Here's how the part is built. I have some questions about the finished solid (model axes, mm). Face numbers are marked on the shaded views. A direction names the side the tool comes from. Round coordinates to 2 decimals unless told otherwise and drop trailing zeros. Loops run counter-clockwise (first coordinate to the right, second up) from the corner with the lowest first, then second, coordinate; pieces in that order, holes last. Notation, with made-up numbers: (62, -11.5) - (79, -11.5) arc R29 ccw to (79, 15.5) - close; hole circle Ø1 at (-40, -23). An arc over 180 degrees is marked (long way). Return JSON: item names as keys, results as strings. Group by question number.
```python
from build123d import *

# Parameters (mm, degrees)
F0_W      = 37
F0_H      = 15
F1_DEPTH  = 3.97
F2_W      = 17
F2_H      = 13.5
F3_DEPTH  = 13.5
F4_R      = 4.85
F5_DEPTH  = 15
F6_R      = 3.15
F7_DEPTH  = 22.001
F8_W      = 17
F8_H      = 7
F9_DEPTH  = 9
F10_R     = 1.55
F11_DEPTH = 11.001
F12_W     = 17
F12_H     = 3
F13_DEPTH = 17.5
F15_DEPTH = 3.971


with BuildPart() as f1:
    # F0 (on Top) → F1 (new body)
    with BuildSketch(Plane.XY):
        Rectangle(F0_W, F0_H)
    extrude(amount=F1_DEPTH)

    # F2 (on face) → F3 (join)
    with BuildSketch(Plane.XY.offset(3.97)):
        with Locations((-10, 0)):
            Rectangle(F2_W, F2_H)
    extrude(amount=F3_DEPTH)

    # F4 (on face) → F5 (cut)
    with BuildSketch(Plane(origin=(-18.5, 0, 0), x_dir=(0, -1, 0), z_dir=(-1, 0, 0))):
        with Locations((0, 8.82)):
            Circle(F4_R)
    extrude(amount=-F5_DEPTH, mode=Mode.SUBTRACT)

    # F6 (on face) → F7 (cut, through all)
    with BuildSketch(Plane(origin=(-3.5, 0, 0), x_dir=(0, -1, 0), z_dir=(-1, 0, 0))):
        with Locations((0, 8.82)):
            Circle(F6_R)
    extrude(amount=-F7_DEPTH, mode=Mode.SUBTRACT)

    # F8 (on face) → F9 (join)
    with BuildSketch(Plane.XY.offset(17.47)):
        with Locations((-10, 0)):
            Rectangle(F8_W, F8_H)
    extrude(amount=F9_DEPTH)

    # F10 (on face) → F11 (cut, through all)
    with BuildSketch(Plane.XZ.offset(3.5)):
        with Locations((-10, 21.97)):
            Circle(F10_R)
    extrude(amount=-F11_DEPTH, mode=Mode.SUBTRACT)

    # F12 (on face) → F13 (cut)
    with BuildSketch(Plane.XY.offset(26.47)):
        with Locations((-10, 0)):
            Rectangle(F12_W, F12_H)
    extrude(amount=-F13_DEPTH, mode=Mode.SUBTRACT)

    # F14 (on face) → F15 (cut, through all)
    with BuildSketch(Plane.XY.offset(3.97)):
        with BuildLine():
            Line((14.45, 5.8), (4.45, 5.8))
            ThreePointArc((4.45, 5.8), (2.8, 4.15), (4.45, 2.5))
            Line((4.45, 2.5), (14.45, 2.5))
            ThreePointArc((14.45, 2.5), (16.1, 4.15), (14.45, 5.8))
        make_face()
        with BuildLine():
            Line((14.45, -2.5), (4.45, -2.5))
            ThreePointArc((4.45, -2.5), (2.8, -4.15), (4.45, -5.8))
            Line((4.45, -5.8), (14.45, -5.8))
            ThreePointArc((14.45, -5.8), (16.1, -4.15), (14.45, -2.5))
        make_face()
    extrude(amount=-F15_DEPTH, mode=Mode.SUBTRACT)


solid = f1.part
```
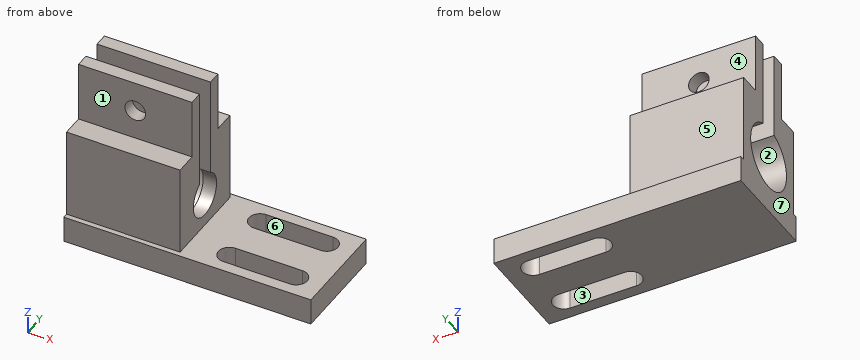
Q1. Will these pins go through, and if not, where does the flat tip stop? pin 1 Ø12 at (x, z) = (-4, 15) entering from +Y; pin 2 Ø5 at (x, z) = (-14, 11.5) entering from -Y; pin 3 Ø3 at (y, z) = (3, 9) entering from +X.
Q2. Imagine slicing it at A-A, the plane z = 8.82. List the corners of the cut face in (x, y) for me.
Q3. Imagine slicing it at D-D, the plane z = 21.97. List the corners of the cut face in (x, y) for me.
Q4. For the marked faces 1, 2, 3 and 4, which set-ups out of +Z, -Z, +X, -X, +Y, -Y let a thin tool reach every point of the face, with its end or its side?
Q5. Please list where these lines run through material, in increasing order: line 1 (Z direction, x = -10, y = 2); line 2 (Z direction, x = -10, y = 2.8); line 3 (Y direction, x = -12.5, z = 16.5).
Q6. Imagine slicing it at B-B, the plane x = -10. List the corners of the cut face in (y, z) for me, and give its area (3 significant figures).
Q7. Imagine slicing it at C-C, the plane y = 0. List the corners of the cut face in (x, z) for me.
Q8. If we mould it in two halves opening along X, with no side actions, what happens to the marked faces 5, 6 and 7? For each: +X half, -X half, draft (parallel to the pull), parting line (faces both ways), or undercut.
Output values:
{
 "1": {"pin 1": "stops at y = 6.75", "pin 2": "stops at y = -6.75", "pin 3": "stops at x = -1.5"},
 "2": {"outline": "(-18.5, -6.75) - (-1.5, -6.75) - (-1.5, -3.15) - (-3.5, -3.15) - (-3.5, -4.85) - (-18.5, -4.85) - close; (-18.5, 4.85) - (-3.5, 4.85) - (-3.5, 3.15) - (-1.5, 3.15) - (-1.5, 6.75) - (-18.5, 6.75) - close"},
 "3": {"outline": "(-18.5, -3.5) - (-11.55, -3.5) - (-11.55, -1.5) - (-18.5, -1.5) - close; (-18.5, 1.5) - (-11.55, 1.5) - (-11.55, 3.5) - (-18.5, 3.5) - close; (-8.45, -3.5) - (-1.5, -3.5) - (-1.5, -1.5) - (-8.45, -1.5) - close; (-8.45, 1.5) - (-1.5, 1.5) - (-1.5, 3.5) - (-8.45, 3.5) - close"},
 "4": {"face 1": "+Z, +X, -X, -Y", "face 2": "-X", "face 3": "+Z, -Z", "face 4": "+Z, +X, -X, +Y"},
 "5": {"line 1": "z = 0 to 4.4, 13.24 to 20.42, 23.52 to 26.47", "line 2": "z = 0 to 4.86, 12.78 to 20.42, 23.52 to 26.47", "line 3": "y = -6.75 to -1.5, 1.5 to 6.75"},
 "6": {"outline": "(-7.5, 0) - (7.5, 0) - (7.5, 3.97) - (6.75, 3.97) - (6.75, 17.47) - (3.5, 17.47) - (3.5, 20.42) - (1.5, 20.42) - (1.5, 13.43) arc R4.85 cw (long way) to (-1.5, 13.43) - (-1.5, 20.42) - (-3.5, 20.42) - (-3.5, 17.47) - (-6.75, 17.47) - (-6.75, 3.97) - (-7.5, 3.97) - close; (-3.5, 23.52) - (-1.5, 23.52) - (-1.5, 26.47) - (-3.5, 26.47) - close; (1.5, 23.52) - (3.5, 23.52) - (3.5, 26.47) - (1.5, 26.47) - close", "area": "180 mm^2"},
 "7": {"outline": "(-18.5, 0) - (18.5, 0) - (18.5, 3.97) - (-1.5, 3.97) - (-1.5, 5.67) - (-3.5, 5.67) - (-3.5, 3.97) - (-18.5, 3.97) - close"},
 "8": {"face 5": "draft", "face 6": "undercut", "face 7": "-X half"}
}
